Build history of the part. All positions in model axes, mm. Face numbers are marked on the shaded views. A direction names the side the tool comes from. Give positions to 0.01 mm unless a question says otherwise; leave off trailing zeros. Loops run counter-clockwise (first coordinate to the right, second up) from the corner with the lowest first, then second, coordinate; pieces in that order, holes last. Notation, with made-up numbers: M 84,1 L 102,1 A11 cw 102,21 Z; hole C -25.5,57.25 d6. An arc over 180 degrees is marked long. Put each result on its own line as item: value.
```python
from build123d import *

# Parameters (mm, degrees)
ESBO_O1_R                = 9
RESSALTO_EXTRUS_O1_DEPTH = 11
ESBO_O2_R                = 9
ESBO_O2_R_2              = 7.5
CORTE_EXTRUS_O1_DEPTH    = 12
ESBO_O3_R                = 3
CORTE_EXTRUS_O2_DEPTH    = 16
CORTE_EXTRUS_O3_REACH    = 27.417
ESBO_O4_R                = 2.1
ESBO_O8_R                = 1.65
CORTE_EXTRUS_O4_DEPTH    = 17.822603841


with BuildPart() as part:
    # Esboço1 → Ressalto-extrusão1 (new, symmetric)
    with BuildSketch(Plane(origin=(0, 0, 0), x_dir=(0, 0, -1), z_dir=(1, 0, 0))):
        Circle(ESBO_O1_R)
    extrude(amount=RESSALTO_EXTRUS_O1_DEPTH, both=True)

    # Esboço2 → Corte-extrusão1 (cut)
    with BuildSketch(Plane(origin=(11, 0, 0), x_dir=(0, 0, -1), z_dir=(1, 0, 0))):
        Circle(ESBO_O2_R)
        Circle(ESBO_O2_R_2, mode=Mode.SUBTRACT)
    extrude(amount=-CORTE_EXTRUS_O1_DEPTH, mode=Mode.SUBTRACT)

    # Esboço3 → Corte-extrusão2 (cut)
    with BuildSketch(Plane(origin=(11, 0, 0), x_dir=(0, 0, -1), z_dir=(1, 0, 0))):
        Circle(ESBO_O3_R)
    extrude(amount=-CORTE_EXTRUS_O2_DEPTH, mode=Mode.SUBTRACT)

    # Esboço4 → Corte-extrusão3 (cut, up to next)
    with BuildSketch(Plane.ZY.offset(11), mode=Mode.PRIVATE) as corte_extrus_o3_sk1:
        Circle(ESBO_O4_R)
    corte_extrus_o3_tool1 = extrude(corte_extrus_o3_sk1.sketch, amount=-CORTE_EXTRUS_O3_REACH, mode=Mode.PRIVATE) & part.part
    add(corte_extrus_o3_tool1.solids().sort_by_distance((-11, 0, 0))[0], mode=Mode.SUBTRACT)

    # Esboço8 → Corte-extrusão4 (cut, through all)
    with BuildSketch(Plane(origin=(0, 0, 0), x_dir=(1, 0, 0), z_dir=(0, 1, 0))):
        with Locations(Location((5, 0, 0), (0, 0, 90))):
            Circle(ESBO_O8_R)
    extrude(amount=CORTE_EXTRUS_O4_DEPTH, mode=Mode.SUBTRACT)


solid = part.part
```
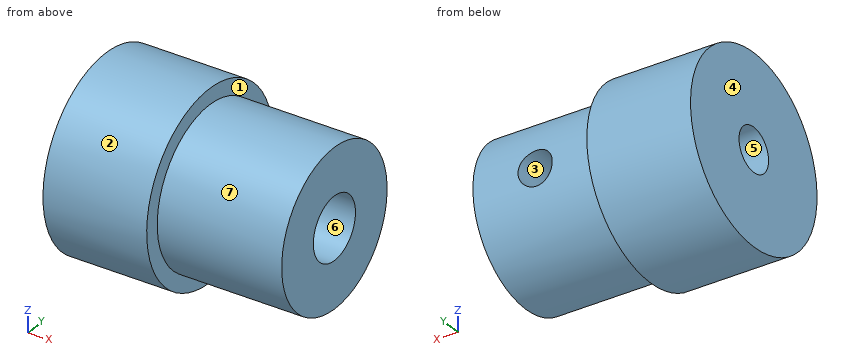
Q1. Slice it at D-D (x = -2.5). List the corners of the cut face in (y, z), and give its area (3 significant figures).
Here are the results:
outline: C 0,0 d18; hole C 0,0 d6
area: 226 mm²
Q2. Tool access for the marked faces 1, 2 and 3: list every direction of +Z, -Z, +X, -X, +Y, -Y with a clear straight run to the whole face (end or side of a thin tool).
Here are the results:
face 1: +X
face 2: +X, -X
face 3: +Y
Q3. Slice it at A-A (z = 0). List the corners of the cut face in (x, y), and give its area (3 significant figures).
Here are the results:
outline: M -11,-9 L -1,-9 L -1,-7.5 L 11,-7.5 L 11,-3 L -5,-3 L -5,-2.1 L -11,-2.1 Z; M -11,2.1 L -5,2.1 L -5,3 L 3.35,3 L 3.35,7.5 L -1,7.5 L -1,9 L -11,9 Z; M 6.65,3 L 11,3 L 11,7.5 L 6.65,7.5 Z
area: 224 mm²
Q4. Drop flat-ended pins along their axis: pin 1 Ø1 at (x, y) = (6, -6) entering from -Z; pin 2 Ø3 at (y, z) = (0.5, -1) entering from +X; pin 3 Ø1 at (x, y) = (-2.5, 1.5) entering from -Z. Give the stop position or say it passes through.
Here are the results:
pin 1: z = -5.1
pin 2: x = -5
pin 3: z = -8.94
Q5. Slice it at C-C (y = -4.25). List the corners of the cut face in (x, z).
Here are the results:
outline: M -11,-7.93 L -1,-7.93 L -1,-6.18 L 11,-6.18 L 11,6.18 L -1,6.18 L -1,7.93 L -11,7.93 Z
Q6. Slice it at B-B (y = 0). List the corners of the cut face in (x, z), and give its area (3 significant figures).
Here are the results:
outline: M -11,-9 L -1,-9 L -1,-7.5 L 11,-7.5 L 11,-3 L -5,-3 L -5,-2.1 L -11,-2.1 Z; M -11,2.1 L -5,2.1 L -5,3 L 11,3 L 11,7.5 L -1,7.5 L -1,9 L -11,9 Z
area: 239 mm²
Q7. Mould opens along Y. For the marked faces 4, 5, 6 and 7 say: pulls with the +Y half, pulls with the -Y half, needs draft (parallel to the pull), parting line crosses it, or undercut.
Here are the results:
face 4: needs draft
face 5: undercut
face 6: undercut
face 7: parting line crosses it
Q8. Probe line 1 (Y direction, x = 7.25, z = 0); line 2 (X direction, y = 4.5, z = 0); line 3 (Y direction, x = -5.75, z = -0.75). List the from-to ranges inside material, lowest first. Write a range as from..to.
Here are the results:
line 1: -7.5..-3, 3..7.5
line 2: -11..3.35, 6.65..11
line 3: -8.97..-1.96, 1.96..8.97
